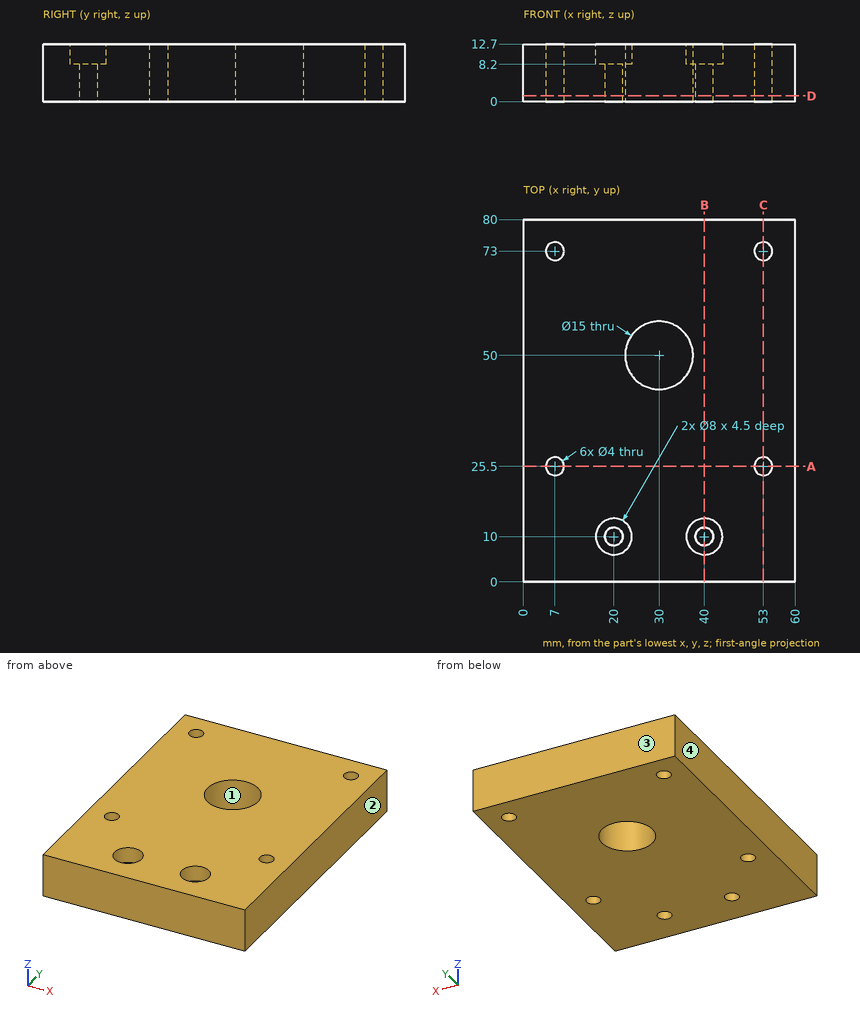
Input: dimensioned drawing with shaded views. Units: mm. Origin: part minimum x, y, z. Coordinates: 2 decimals unless noted, no trailing zeros. Order: outer loops, then holes, each group sorted by start corner. A loop starts at its lowest first (then second) coordinate and runs counter-clockwise, first axis right, second up. Notation, with made-up numbers: (-38.5, 86.5) -> (-17.5, 86.5) arc R5 ccw to (-17.5, 92.5) -> close; hole circle Ø6 at (-26.5, 69). An arc over 180 degrees is marked (long way). Use CSV: the item, a comma, the result in double quotes.
1) Section B-B on x = 40. Output: boundary loops of the cut face in (y, z).
Findings:
outline,"(0, 0) -> (8, 0) -> (8, 8.2) -> (6, 8.2) -> (6, 12.7) -> (0, 12.7) -> close; (12, 0) -> (80, 0) -> (80, 12.7) -> (14, 12.7) -> (14, 8.2) -> (12, 8.2) -> close"
2) Line query: line 1 (Y direction, x = 53, z = 9.25); line 2 (X direction, y = 73, z = 9); line 3 (X direction, y = 10, z = 5.5). Output: solid intervals per line, ascending.
Findings:
line 1,"y = 0 to 23.5, 27.5 to 71, 75 to 80"
line 2,"x = 0 to 5, 9 to 51, 55 to 60"
line 3,"x = 0 to 18, 22 to 38, 42 to 60"
3) Mould query, pull axis X, two halves, no side actions, for the marked faces 1, 2, 3 and 4. Classes: +X half, -X half, draft (parallel to the pull), parting line (faces both ways), or undercut.
Findings:
face 1,"undercut"
face 2,"+X half"
face 3,"draft"
face 4,"-X half"
4) Section A-A on y = 25.5. Output: boundary loops of the cut face in (x, z).
Findings:
outline,"(0, 0) -> (5, 0) -> (5, 12.7) -> (0, 12.7) -> close; (9, 0) -> (51, 0) -> (51, 12.7) -> (9, 12.7) -> close; (55, 0) -> (60, 0) -> (60, 12.7) -> (55, 12.7) -> close"
5) Section D-D on z = 1.25. Output: boundary loops of the cut face in (x, y), then the cut area to 3 significant figures.
Findings:
outline,"(0, 0) -> (60, 0) -> (60, 80) -> (0, 80) -> close; hole circle Ø4 at (7, 25.5); hole circle Ø4 at (7, 73); hole circle Ø4 at (20, 10); hole circle Ø15 at (30, 50); hole circle Ø4 at (40, 10); hole circle Ø4 at (53, 25.5); hole circle Ø4 at (53, 73)"
area,"4,550 mm^2"
6) Section C-C on x = 53. Output: boundary loops of the cut face in (y, z), then the cut area to 3 significant figures.
Findings:
outline,"(0, 0) -> (23.5, 0) -> (23.5, 12.7) -> (0, 12.7) -> close; (27.5, 0) -> (71, 0) -> (71, 12.7) -> (27.5, 12.7) -> close; (75, 0) -> (80, 0) -> (80, 12.7) -> (75, 12.7) -> close"
area,"914 mm^2"
7) Pin query (flat end, axial travel): pin 1 Ø4.5 at (x, y) = (40, 10) entering from +Z; pin 2 Ø4.5 at (x, y) = (7, 73) entering from -Z; pin 3 Ø2.5 at (x, y) = (53, 73) entering from +Z. Return the tip coordinate at first contact, or that it passes through.
Findings:
pin 1,"stops at z = 8.2"
pin 2,"stops at z = 0"
pin 3,"passes through"
